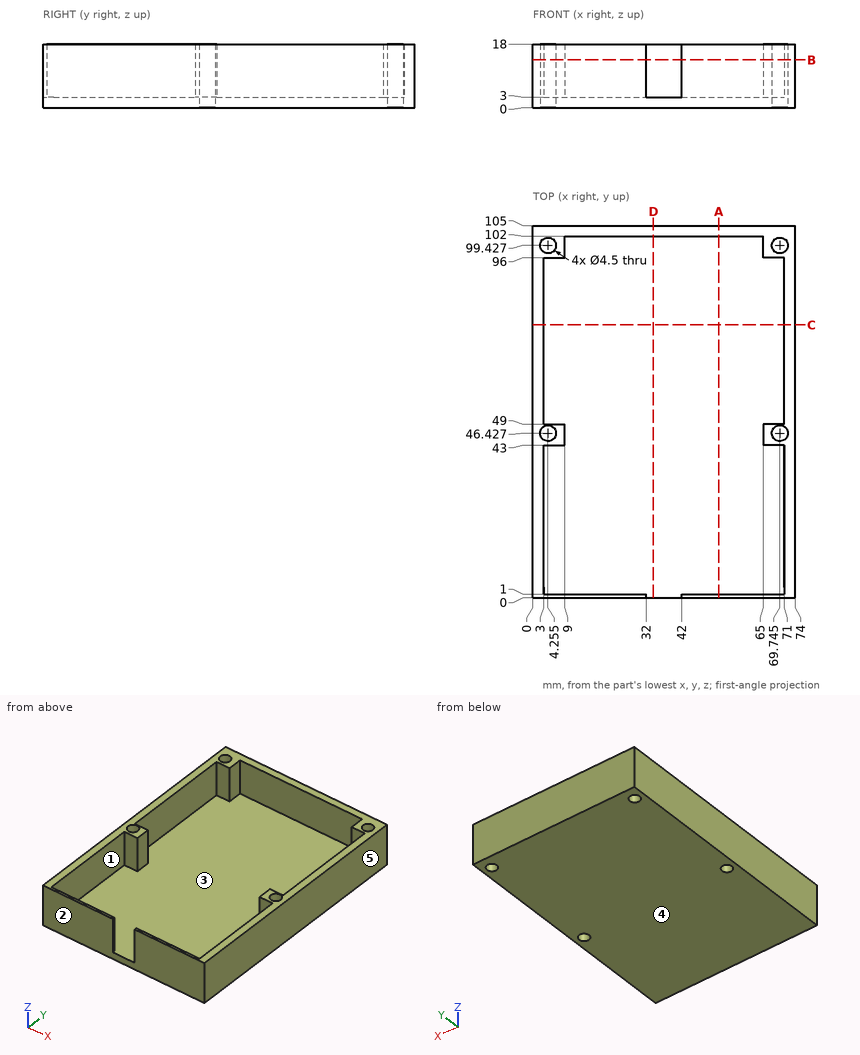
Part print with two shaded views. Sizes in mm from the minimum x, y, z corner. A direction names the side the tool comes from. Round coordinates to 2 decimals unless told otherwise and drop trailing zeros. Write each loop counter-clockwise with the first axis right and the second up, starting at its lowest first coordinate (ties: lowest second). Pieces come first, ordered by that corner, then holes. Notation, with made-up numbers: (84, -8.5) - (93, -8.5) arc R20 ccw to (93, 17.5) - close; hole circle Ø10 at (27.5, 17.25). An arc over 180 degrees is marked (long way). Answer as CSV lines item,"result".
Q1. Cut at B-B (z = 13.5). State how many separate pieces and enclosed holes the cut face has.
Report:
separate pieces,"1"
enclosed holes,"4"
Q2. Cut at C-C (y = 77). Write the cut outline in (x, z), and give its area (3 significant figures).
Report:
outline,"(0, 0) - (74, 0) - (74, 18) - (71, 18) - (71, 3) - (3, 3) - (3, 18) - (0, 18) - close"
area,"312 mm^2"
Q3. Drill centre lines: probe 1 along Y at (x, z) = (53, 10.75); probe 2 along Y at (x, z) = (69, 12.5); probe 3 along X at (y, z) = (70, 4.5). Where is each one in solid material? Low to high. Write a range as [from, to].
Report:
probe 1,"y = [0, 1], [102, 105]"
probe 2,"y = [0, 1], [43, 44.3], [48.55, 49], [96, 97.3], [101.55, 105]"
probe 3,"x = [0, 3], [71, 74]"
Q4. Cut at D-D (x = 34). Write the cut outline in (y, z).
Report:
outline,"(0, 0) - (105, 0) - (105, 18) - (102, 18) - (102, 3) - (0, 3) - close"
Q5. Pull direction X, two halves, no side cores. Call the marked faces 3, 4 and 5: +X half, -X half, draft (parallel to the pull), parting line (faces both ways), or undercut.
Report:
face 3,"undercut"
face 4,"draft"
face 5,"+X half"
Q6. Cut at A-A (x = 52.5). Write the cut outline in (y, z), and give its area (3 significant figures).
Report:
outline,"(0, 0) - (105, 0) - (105, 18) - (102, 18) - (102, 3) - (1, 3) - (1, 18) - (0, 18) - close"
area,"375 mm^2"
Q7. Drop a flat-ended pin along its axis: pin 1 (8 mm diameter, centred on x = 59.5, y = 58.5, fed in from +Z). Give the stop position or say it passes through.
Report:
pin 1,"stops at z = 3"
Q8. Tool access for the marked faces 1 and 2: list every direction of +Z, -Z, +X, -X, +Y, -Y with a clear straight run to the whole face (end or side of a thin tool).
Report:
face 1,"+Z"
face 2,"+Z, -Z, +X, -X, -Y"
